Verification items for the finished model (mm, model axes). Give positions to 0.01 mm unless a question says otherwise; leave off trailing zeros. Loops run counter-clockwise (first coordinate to the right, second up) from the corner with the lowest first, then second, coordinate; pieces in that order, holes last. Notation, with made-up numbers: (71.25, -1.5) -> (96.25, -1.5) arc R15 ccw to (96.25, 25.5) -> close; hole circle Ø3 at (45, -21). An arc over 180 degrees is marked (long way). Answer in a Markdown table with one row per item. Add a question column.
Q1. Gauge pin test, flat end, axial feed: P1, Ø3, axis at x = 2.5, y = -0.5, coming from the -Z side. Record the tip position at first contact, or that the pin passes through.
Q2. Section check A-A on z = 0.15. Enter the section's corners in (x, y), and give its area (3 significant figures).
Q3. Material ranges on probe 1 along X at (y, z) = (-5.5, 0.05); probe 2 along Y at (x, z) = (-7.75, 0.1); probe 3 along X at (y, z) = (-0.25, 0.25), recorded low to high.
```python
from build123d import *

# Parameters (mm, degrees)
PAD_DEPTH = 0.3
FILLET_R  = 0.29


with BuildPart() as part:
    # Sketch → Pad (new body)
    with BuildSketch(Plane.XY):
        with BuildLine():
            Line((-8, 7.5), (8, 7.5))
            ThreePointArc((10, 5.5), (9.414214, 6.914214), (8, 7.5))
            Line((10, 5.5), (10, -5.5))
            ThreePointArc((8, -7.5), (9.414214, -6.914214), (10, -5.5))
            Line((8, -7.5), (-8, -7.5))
            ThreePointArc((-10, -5.5), (-9.414214, -6.914214), (-8, -7.5))
            Line((-10, -5.5), (-10, 5.5))
            ThreePointArc((-8, 7.5), (-9.414214, 6.914214), (-10, 5.5))
        make_face()
    extrude(amount=PAD_DEPTH)

    # Fillet
    fillet_edges = [part.edges().sort_by_distance(p)[0] for p in [
        (0, 7.5, 0.3),
        (-9.414214, 6.914214, 0.3),
        (-10, 0, 0.3),
        (-9.414214, -6.914214, 0.3),
        (0, -7.5, 0.3),
        (9.414214, -6.914214, 0.3),
        (10, 0, 0.3),
        (9.414214, 6.914214, 0.3),
    ]]
    fillet(fillet_edges, radius=FILLET_R)


solid = part.part
```
Taken from the geometry:
| question | item | result |
|---|---|---|
| 1 | P1 | stops at z = 0 |
| 2 | outline | (-9.96, -5.5) arc R1.96 ccw to (-8, -7.46) -> (8, -7.46) arc R1.96 ccw to (9.96, -5.5) -> (9.96, 5.5) arc R1.96 ccw to (8, 7.46) -> (-8, 7.46) arc R1.96 ccw to (-9.96, 5.5) -> close |
| 2 | area | 294 mm² |
| 3 | probe 1 | x = -10 to 10 |
| 3 | probe 2 | y = -7.49 to 7.49 |
| 3 | probe 3 | x = -9.87 to 9.87 |
